```python
from build123d import *

# Parameters (mm, degrees)
SKETCH_1_W          = 228
SKETCH_1_H          = 84
SKETCH_1_R          = 2.15
EXTRUDE_1_DEPTH     = 1
SKETCH_3_R          = 1.7
SKETCH_3_R_2        = 1.6
SKETCH_3_R_3        = 4
CUT_EXTRUDE_1_DEPTH = 10
SKETCH_4_R          = 3.5
SKETCH_4_R_2        = 8
CUT_EXTRUDE_2_DEPTH = 1


with BuildPart() as part:
    # Эскиз1 → Вытянуть1 (new body)
    with BuildSketch(Plane.XY):
        Rectangle(SKETCH_1_W, SKETCH_1_H)
        with Locations((107, 32)):
            Circle(SKETCH_1_R, mode=Mode.SUBTRACT)
        with Locations(Location((-107, 32, 0), (0, 0, 180))):
            Circle(SKETCH_1_R, mode=Mode.SUBTRACT)
        with Locations((-107, -32)):
            Circle(SKETCH_1_R, mode=Mode.SUBTRACT)
        with Locations(Location((107, -32, 0), (0, 0, 180))):
            Circle(SKETCH_1_R, mode=Mode.SUBTRACT)
    extrude(amount=EXTRUDE_1_DEPTH)

    # Эскиз3 → Вырез-Вытянуть1 (cut)
    with BuildSketch(Plane.XY.offset(1)):
        with Locations((37, -22)):
            Circle(SKETCH_3_R)
        with Locations((84, -22)):
            Circle(SKETCH_3_R)
        with Locations((38.5, 17)):
            Circle(SKETCH_3_R_2)
        with Locations((82.5, 17)):
            Circle(SKETCH_3_R_2)
        with Locations((51.5, 22)):
            Circle(SKETCH_3_R_3)
        with Locations((69.5, 22)):
            Circle(SKETCH_3_R_3)
        with BuildLine():
            Line((40.14870942, -25.864196381), (40.875982147, -17.864196381))
            ThreePointArc((40.875982147, -17.864196381), (41.358314525, -16.892366164), (42.369821957, -16.5))
            Line((42.369821957, -16.5), (78.630178043, -16.5))
            ThreePointArc((78.630178043, -16.5), (79.641685475, -16.892366164), (80.124017853, -17.864196381))
            Line((80.124017853, -17.864196381), (80.85129058, -25.864196381))
            ThreePointArc((80.85129058, -25.864196381), (80.465084606, -27.011507432), (79.35745077, -27.5))
            Line((79.35745077, -27.5), (41.64254923, -27.5))
            ThreePointArc((41.64254923, -27.5), (40.534915394, -27.011507432), (40.14870942, -25.864196381))
        make_face()
    extrude(amount=-CUT_EXTRUDE_1_DEPTH, mode=Mode.SUBTRACT)

    # Эскиз4 → Вырез-Вытянуть2 (cut)
    with BuildSketch(Plane.XY.offset(1)):
        with Locations((-108, 9)):
            Circle(SKETCH_4_R)
        with Locations((-64, -17)):
            Circle(SKETCH_4_R_2)
    extrude(amount=-CUT_EXTRUDE_2_DEPTH, mode=Mode.SUBTRACT)


solid = part.part
```
CAD build for the part. Positions are in the model's coordinates, mm. Coordinates: 2 decimals unless noted, no trailing zeros. Loops run counter-clockwise (first coordinate to the right, second up) from the corner with the lowest first, then second, coordinate; pieces in that order, holes last. Notation, with made-up numbers: (-2.75, 55) - (52.25, 55) arc R15 ccw to (52.25, 81) - close; hole circle Ø1 at (70.5, 39.5). An arc over 180 degrees is marked (long way). Return JSON: item names as keys, results as strings.
1. Probe L1, parallel to Y at x = 52, z = 0.7; L2, parallel to Y at x = -64, z = 0.75; L3, parallel to X at y = -31, z = 0.7. List the from-to ranges inside material, lowest first. Write a range as from..to.
Result:
{"L1": "y = -42..-27.5, -16.5..18.03, 25.97..42", "L2": "y = -42..-25, -9..42", "L3": "x = -114..-108.9, -105.1..105.1, 108.9..114"}
2. Band-saw the part on A-A (y = 9). Give the cut face in (x, z), and give its area (3 significant figures).
Result:
{"outline": "(-114, 0) - (-111.5, 0) - (-111.5, 1) - (-114, 1) - close; (-104.5, 0) - (114, 0) - (114, 1) - (-104.5, 1) - close", "area": "221 mm2"}
3. Band-saw the part on C-C (y = 32). Give the cut face in (x, z).
Result:
{"outline": "(-114, 0) - (-109.15, 0) - (-109.15, 1) - (-114, 1) - close; (-104.85, 0) - (104.85, 0) - (104.85, 1) - (-104.85, 1) - close; (109.15, 0) - (114, 0) - (114, 1) - (109.15, 1) - close"}
4. Mould opens along X. For faces 1 (the cylindrical face through (-104.767, 7.659, 0.507)), 2 (the flat face through (-2, 1, 1)) say: released by +X, released by -X, zero draft, split by the parting line, or undercut.
Result:
{"face 1": "undercut", "face 2": "zero draft"}
5. Band-saw the part on B-B (x = 107). Give the cut face in (y, z), and give its area (3 significant figures).
Result:
{"outline": "(-42, 0) - (-34.15, 0) - (-34.15, 1) - (-42, 1) - close; (-29.85, 0) - (29.85, 0) - (29.85, 1) - (-29.85, 1) - close; (34.15, 0) - (42, 0) - (42, 1) - (34.15, 1) - close", "area": "75.4 mm2"}
6. Band-saw the part on D-D (x = -64). Give the cut face in (y, z).
Result:
{"outline": "(-42, 0) - (-25, 0) - (-25, 1) - (-42, 1) - close; (-9, 0) - (42, 0) - (42, 1) - (-9, 1) - close"}
